```python
from build123d import *

# Parameters (mm, degrees)
F1_DEPTH = 19.05
F3_DEPTH = 25.4


with BuildPart() as f1:
    # F0 (on Front) → F1 (new body)
    with BuildSketch(Plane.XZ):
        with BuildLine():
            Line((20.027097595, 36.4074036121), (2.6105293283, 42.9636023111))
            ThreePointArc((2.6105293283, 42.9636023111), (16.9814393634, 23.5834144733), (22.0743066938, 0))
            ThreePointArc((22.0743066938, 0), (16.9814393634, -23.5834144733), (2.6105293283, -42.9636023111))
            Line((2.6105293283, -42.9636023111), (20.027097595, -36.4074036121))
            ThreePointArc((20.027097595, -36.4074036121), (24.4278254251, -35.189367606), (28.975523916, -34.7789341976))
            Line((28.975523916, -34.7789341976), (59.6230894717, -34.7789341976))
            ThreePointArc((59.6230894717, -34.7789341976), (64.1707879626, -35.189367606), (68.5715157927, -36.4074036121))
            Line((68.5715157927, -36.4074036121), (85.9880840594, -42.9636023111))
            ThreePointArc((85.9880840594, -42.9636023111), (66.5243066938, 0), (85.9880840594, 42.9636023111))
            Line((85.9880840594, 42.9636023111), (68.5715157927, 36.4074036121))
            ThreePointArc((68.5715157927, 36.4074036121), (64.1707879626, 35.189367606), (59.6230894717, 34.7789341976))
            Line((59.6230894717, 34.7789341976), (28.975523916, 34.7789341976))
            ThreePointArc((28.975523916, 34.7789341976), (24.4278254251, 35.189367606), (20.027097595, 36.4074036121))
        make_face()
        with BuildLine():
            ThreePointArc((2.6105293283, 42.9636023111), (-14.941734084, 53.4859438174), (-35.0756933062, 57.15))
            Line((-35.0756933062, 57.15), (2.6105293283, 42.9636023111))
        make_face()
        with BuildLine():
            Line((123.6743066938, 57.15), (85.9880840594, 42.9636023111))
            ThreePointArc((85.9880840594, 42.9636023111), (66.5243066938, 0), (85.9880840594, -42.9636023111))
            Line((85.9880840594, -42.9636023111), (123.6743066938, -57.15))
            ThreePointArc((123.6743066938, -57.15), (164.0854592386, -40.4111525448), (180.8243066938, 0))
            ThreePointArc((180.8243066938, 0), (164.0854592386, 40.4111525448), (123.6743066938, 57.15))
        make_face()
        with BuildLine():
            ThreePointArc((123.6743066938, 57.15), (103.5403474717, 53.4859438174), (85.9880840594, 42.9636023111))
            Line((85.9880840594, 42.9636023111), (123.6743066938, 57.15))
        make_face()
        with BuildLine():
            Line((2.6105293283, 42.9636023111), (-35.0756933062, 57.15))
            ThreePointArc((-35.0756933062, 57.15), (-92.2256933062, 0), (-35.0756933062, -57.15))
            Line((-35.0756933062, -57.15), (2.6105293283, -42.9636023111))
            ThreePointArc((2.6105293283, -42.9636023111), (16.9814393634, -23.5834144733), (22.0743066938, 0))
            ThreePointArc((22.0743066938, 0), (16.9814393634, 23.5834144733), (2.6105293283, 42.9636023111))
        make_face()
        with BuildLine():
            Line((2.6105293283, -42.9636023111), (-35.0756933062, -57.15))
            ThreePointArc((-35.0756933062, -57.15), (-14.941734084, -53.4859438174), (2.6105293283, -42.9636023111))
        make_face()
        with BuildLine():
            Line((123.6743066938, -57.15), (85.9880840594, -42.9636023111))
            ThreePointArc((85.9880840594, -42.9636023111), (103.5403474717, -53.4859438174), (123.6743066938, -57.15))
        make_face()
    extrude(amount=F1_DEPTH)

    # F2 (on face) → F3 (cut)
    with BuildSketch(Plane.XZ.offset(19.05)):
        with BuildLine():
            ThreePointArc((-4.721551, -23.0268548625), (1.0359587044, -12.1473696358), (3.0243066938, 0))
            ThreePointArc((3.0243066938, 0), (-62.0164616694, 26.9407683632), (-35.0756933062, -38.1))
            Line((-35.0756933062, -38.1), (-35.0756933062, -31.0422573239))
            Line((-35.0756933062, -31.0422573239), (-4.721551, -23.0268548625))
        make_face()
        with BuildLine():
            Line((-35.0756933062, -31.0422573239), (-35.0756933062, -38.1))
            Line((-35.0756933062, -38.1), (-16.5966969086, -33.3187138428))
            ThreePointArc((-16.5966969086, -33.3187138428), (-10.1227486056, -28.7916750254), (-4.721551, -23.0268548625))
            Line((-4.721551, -23.0268548625), (-35.0756933062, -31.0422573239))
        make_face()
        with BuildLine():
            Line((-16.5966969086, -33.3187138428), (-35.0756933062, -38.1))
            ThreePointArc((-35.0756933062, -38.1), (-25.5319256385, -36.8853154888), (-16.5966969086, -33.3187138428))
        make_face()
        with BuildLine():
            Line((52.6924617589, -7.8659448773), (-4.721551, -23.0268548625))
            ThreePointArc((-4.721551, -23.0268548625), (-10.1227486056, -28.7916750254), (-16.5966969086, -33.3187138428))
            Line((-16.5966969086, -33.3187138428), (52.6924617589, -15.3907220811))
            Line((52.6924617589, -15.3907220811), (65.6350776553, -15.3907220811))
            Line((65.6350776553, -15.3907220811), (97.817716181, -27.9829720911))
            ThreePointArc((97.817716181, -27.9829720911), (93.3797600536, -23.1052038265), (89.8493835117, -17.5352380003))
            Line((89.8493835117, -17.5352380003), (65.6350776553, -7.8659448773))
            Line((65.6350776553, -7.8659448773), (65.6350776553, 0))
            Line((65.6350776553, 0), (52.6924617589, 0))
            Line((52.6924617589, 0), (52.6924617589, -7.8659448773))
        make_face()
        with BuildLine():
            Line((11.3188134617, 0), (52.6924617589, 0))
            Line((52.6924617589, 0), (65.6350776553, 0))
            Line((65.6350776553, 0), (77.279799926, 0))
            Line((77.279799926, 0), (77.279799926, 39.6855029616))
            Line((77.279799926, 39.6855029616), (68.5715157927, 36.4074036121))
            ThreePointArc((68.5715157927, 36.4074036121), (64.1707879626, 35.189367606), (59.6230894717, 34.7789341976))
            Line((59.6230894717, 34.7789341976), (28.975523916, 34.7789341976))
            ThreePointArc((28.975523916, 34.7789341976), (24.4278254251, 35.189367606), (20.027097595, 36.4074036121))
            Line((20.027097595, 36.4074036121), (11.3188134617, 39.6855029616))
            Line((11.3188134617, 39.6855029616), (11.3188134617, 0))
        make_face()
        with BuildLine():
            ThreePointArc((161.7743066938, 0), (114.6498835333, 37.0158045518), (89.8493835117, -17.5352380003))
            Line((89.8493835117, -17.5352380003), (123.6743066938, -31.0422573239))
            Line((123.6743066938, -31.0422573239), (123.6743066938, -38.1))
            ThreePointArc((123.6743066938, -38.1), (150.615075057, -26.9407683632), (161.7743066938, 0))
        make_face()
        with BuildLine():
            Line((123.6743066938, -38.1), (97.817716181, -27.9829720911))
            ThreePointArc((97.817716181, -27.9829720911), (109.791605888, -35.4807076922), (123.6743066938, -38.1))
        make_face()
        with BuildLine():
            ThreePointArc((89.8493835117, -17.5352380003), (93.3797600536, -23.1052038265), (97.817716181, -27.9829720911))
            Line((97.817716181, -27.9829720911), (123.6743066938, -38.1))
            Line((123.6743066938, -38.1), (123.6743066938, -31.0422573239))
            Line((123.6743066938, -31.0422573239), (89.8493835117, -17.5352380003))
        make_face()
    extrude(amount=-F3_DEPTH, mode=Mode.SUBTRACT)


solid = f1.part
```
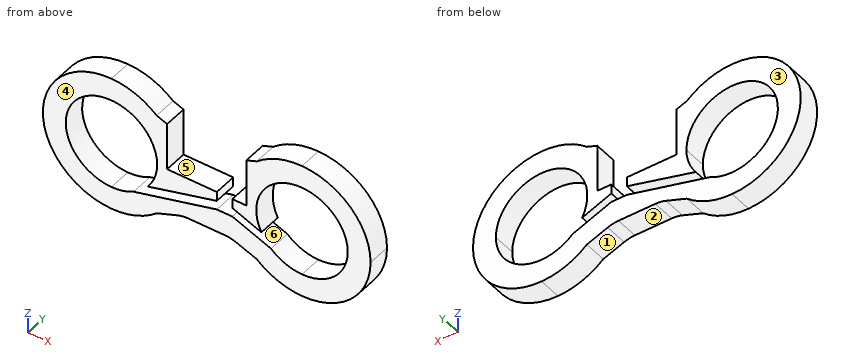
Here's how the part is built. I have some questions about the finished solid (model axes, mm). Face numbers are marked on the shaded views. A direction names the side the tool comes from. Round coordinates to 2 decimals unless told otherwise and drop trailing zeros. Order: outer loops, then holes, each group sorted by start corner. A loop starts at its lowest first (then second) coordinate and runs counter-clockwise, first axis right, second up. Notation, with made-up numbers: M 30.25,-11 L 62.25,-11 A18 ccw 62.25,8 Z; hole C -33,11 d2. An arc over 180 degrees is marked long. Answer in a Markdown table with one row per item.
Item 1: Imagine slicing it at B-B, the plane z = 28. Write out the boundary of the cut face in (x, y).
A:
| item | result |
|---|---|
| outline | M -84.9,-19.05 L -60.91,-19.05 L -60.91,0 L -84.9,0 Z; M -9.24,-19.05 L 11.32,-19.05 L 11.32,0 L -9.24,0 Z; M 77.28,-19.05 L 97.84,-19.05 L 97.84,0 L 77.28,0 Z; M 149.51,-19.05 L 173.5,-19.05 L 173.5,0 L 149.51,0 Z |
Item 2: Imagine slicing it at C-C, the plane y = -7.5. Write out the boundary of the cut face in (x, z), and give its area (3 significant figures).
A:
| item | result |
|---|---|
| outline | M -16.6,-33.32 A38.1 cw long -4.72,-23.03 L 52.69,-7.87 L 52.69,0 L 11.32,0 L 11.32,39.69 L 2.61,42.96 A57.15 ccw long 2.61,-42.96 L 20.03,-36.41 A25.4 cw 28.98,-34.78 L 59.62,-34.78 A25.4 cw 68.57,-36.41 L 85.99,-42.96 A57.15 ccw long 85.99,42.96 L 77.28,39.69 L 77.28,0 L 65.64,0 L 65.64,-7.87 L 89.85,-17.54 A38.1 cw long 97.82,-27.98 L 65.64,-15.39 L 52.69,-15.39 Z |
| area | 12,000 mm2 |
Item 3: If I drill on L1, parallel to X at y = -18, z = -1.5; L2, parallel to X at y = -12.5, z = -4; L3, parallel to Z at x = -59.5, y = -14.5, over which ranges is the centre line in solid material (lowest first)? Write a range as from..to.
A:
| item | result |
|---|---|
| L1 | x = -92.21..-73.15, 2.99..52.69, 65.64..85.6, 161.74..180.8 |
| L2 | x = -92.09..-72.97, 2.81..52.69, 65.64..85.78, 161.56..180.68 |
| L3 | z = -51.67..-29.24, 29.24..51.67 |
Item 4: Imagine slicing it at A-A, the plane x = 37.5. Write out the boundary of the cut face in (y, z), and give its area (3 significant figures).
A:
| item | result |
|---|---|
| outline | M -19.05,-34.78 L 0,-34.78 L 0,-19.32 L -19.05,-19.32 Z; M -19.05,-11.88 L 0,-11.88 L 0,0 L -19.05,0 Z |
| area | 521 mm2 |
Item 5: I'm going to push flat-ended pins straight in: pin 1 (3 mm diameter, centred on y = -12, z = 35, fed in from +X); pin 2 (1 mm diameter, centred on y = -10, z = -18, fed in from +X); pin 3 (3 mm diameter, centred on y = -7, z = -6, fed in from +X). Where does each tip first touch, or does it pass through?
A:
| item | result |
|---|---|
| pin 1 | stops at x = 169.98 |
| pin 2 | stops at x = 178.08 |
| pin 3 | stops at x = 180.65 |
Item 6: Thinking about a two-plate mould opening in X: for the marked faces 1, 2 and 3, which applies, +X half, -X half, draft (parallel to the pull), parting line (faces both ways), or undercut?
A:
| item | result |
|---|---|
| face 1 | undercut |
| face 2 | undercut |
| face 3 | draft |
Item 7: For the marked faces 4, 5 and 6, which set-ups out of +Z, -Z, +X, -X, +Y, -Y let a thin tool reach every point of the face, with its end or its side?
A:
| item | result |
|---|---|
| face 4 | +Z, -Z, +X, -X, -Y |
| face 5 | +Z, +Y, -Y |
| face 6 | +Y, -Y |
Item 8: Imagine slicing it at D-D, the plane x = -24. Write out the boundary of the cut face in (y, z).
A:
| item | result |
|---|---|
| outline | M -19.05,-56.07 L 0,-56.07 L 0,-36.45 L -19.05,-36.45 Z; M -19.05,36.45 L 0,36.45 L 0,56.07 L -19.05,56.07 Z |
